Input: dimensioned drawing with shaded views. Units: mm. Origin: part minimum x, y, z. Coordinates: 2 decimals unless noted, no trailing zeros. Order: outer loops, then holes, each group sorted by start corner. A loop starts at its lowest first (then second) coordinate and runs counter-clockwise, first axis right, second up. Notation, with made-up numbers: (6.5, 74.5) -> (48.5, 74.5) arc R22 cw to (48.5, 81.5) -> close; hole circle Ø2 at (-36, 41). An arc over 180 degrees is marked (long way). Put each result on its own line as item: value.
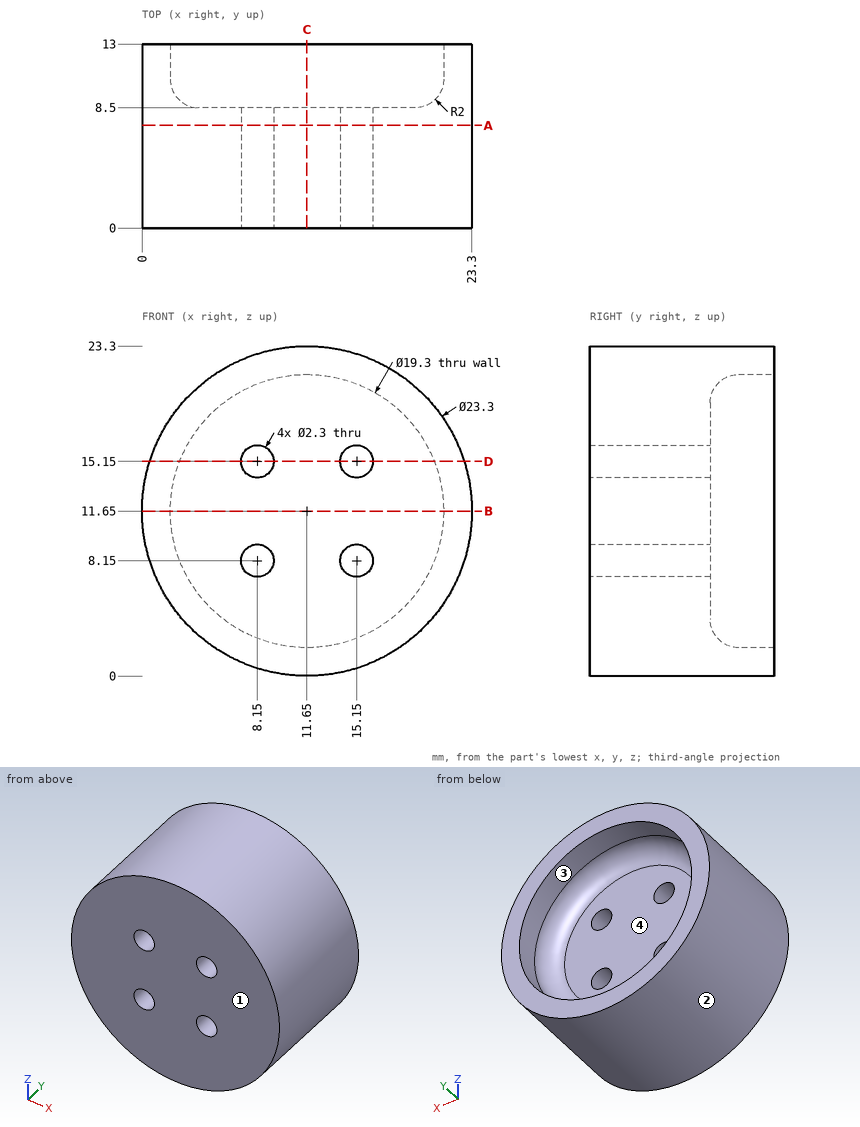
1. Cut plane A-A on y = 7.25. Output: boundary loops of the cut face in (x, z), plus the area to 3 significant figures.
Numbers:
outline: circle Ø23.3 at (11.65, 11.65); hole circle Ø2.3 at (8.15, 8.15); hole circle Ø2.3 at (8.15, 15.15); hole circle Ø2.3 at (15.15, 8.15); hole circle Ø2.3 at (15.15, 15.15)
area: 410 mm2
2. Cut plane C-C on x = 11.65. Output: boundary loops of the cut face in (y, z).
Numbers:
outline: (0, 0) -> (13, 0) -> (13, 2) -> (10.5, 2) arc R2 cw to (8.5, 4) -> (8.5, 19.3) arc R2 cw to (10.5, 21.3) -> (13, 21.3) -> (13, 23.3) -> (0, 23.3) -> close
3. Ray query, line 1 along X through (y, z) = (11.1, 11.65); line 2 along X through (y, z) = (2, 14.5); line 3 along Y through (x, z) = (16.5, 9.75). Return the intervals inside material, ascending.
Numbers:
line 1: x = 0 to 2, 21.3 to 23.3
line 2: x = 0.35 to 7.2, 9.1 to 14.2, 16.1 to 22.95
line 3: y = 0 to 8.5
4. First-contact query: pin 1 (6 mm diameter, centred on y = 10, z = 7, fed in from +X); pin 2 (1.5 mm diameter, centred on x = 13.5, z = 8, fed in from +Y); pin 3 (5 mm diameter, centred on y = 2.5, z = 16.5, fed in from -X). Flat tips, straight axial feed; report the tip coordinate or a pass-through.
Numbers:
pin 1: stops at x = 23.18
pin 2: stops at y = 8.5
pin 3: stops at x = 0.24
5. Pull-direction query (Z, two-part tool) for the marked faces 1, 2, 3 and 4; classes: pulls with the +Z half, pulls with the -Z half, needs draft (parallel to the pull), parting line crosses it, or undercut.
Numbers:
face 1: needs draft
face 2: parting line crosses it
face 3: undercut
face 4: undercut
6. Cut plane B-B on z = 11.65. Output: boundary loops of the cut face in (x, y), plus the area to 3 significant figures.
Numbers:
outline: (0, 0) -> (23.3, 0) -> (23.3, 13) -> (21.3, 13) -> (21.3, 10.5) arc R2 cw to (19.3, 8.5) -> (4, 8.5) arc R2 cw to (2, 10.5) -> (2, 13) -> (0, 13) -> close
area: 218 mm2
7. Cut plane D-D on z = 15.15. Count the separate pieces of the cut face and the enclosed holes in it, plus the area to 3 significant figures.
Numbers:
separate pieces: 3
enclosed holes: 0
area: 171 mm2
